Source: CAD feature listing. Evaluate the final solid. Frame: model axes, mm. Face numbers are marked on the shaded views. A direction names the side the tool comes from. Coordinates: 2 decimals unless noted, no trailing zeros. Write each loop counter-clockwise with the first axis right and the second up, starting at its lowest first coordinate (ties: lowest second). Pieces come first, ordered by that corner, then holes. Notation, with made-up numbers: M 79.5,-8 L 122.5,-8 A25 ccw 122.5,19 Z; hole C -7.5,31.5 d2. An arc over 180 degrees is marked long. One line per item, written item: value. Start each with the question number.
Item 1: Cut plane A-A, the plane x = 22. Output: boundary loops of the cut face in (y, z), then the cut area to 3 significant figures.
Item 2: Set-up query: the marked faces 5, 6 and 7. Return all of +Z, -Z, +X, -X, +Y, -Y with unobstructed straight access to the full face (end or side cutting, diameter ignored); none if empty.
Item 3: Mould query, pull axis Y, two halves, no side actions, for the marked faces 1, 2, 3 and 4. Classes: released by +Y, released by -Y, zero draft, split by the parting line, or undercut.
Item 4: Cut plane B-B, the plane y = 35.5. Output: boundary loops of the cut face in (x, z), then the cut area to 3 significant figures.
Item 5: Cut plane C-C, the plane z = 5.5. Output: boundary loops of the cut face in (x, y).
Item 6: Cut plane D-D, the plane x = 56.5. Output: boundary loops of the cut face in (y, z), then the cut area to 3 significant figures.
Item 7: Pin query (flat end, axial travel): P1, Ø17, axis at y = 54.5, z = 25, coming from the -X side; P2, Ø17, axis at y = 22.5, z = 24, coming from the +X side; P3, Ø0.9, axis at x = 102.5, z = 25.5, coming from the +Y side. Return the tip coordinate at first contact, or that it passes through.
Item 8: Ray query, L1, parallel to Y at x = 48, z = 27.5; L2, parallel to X at y = 57, z = 17.5; L3, parallel to Y at x = 16, z = 14.5. Return the intervals inside material, ascending. Write a range as from..to.
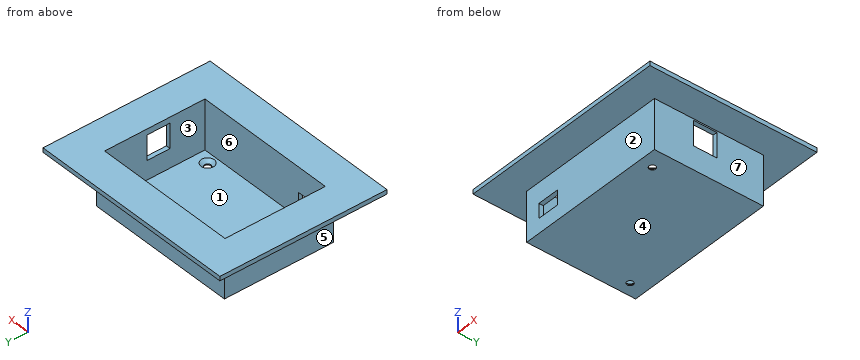
```python
from build123d import *

# Parameters (mm, degrees)
F0_W           = 104
F0_H           = 75
F1_DEPTH       = 37
F2_T           = -3
F4_D           = 4.4
F4_CSINK_D     = 8.96
F4_CSINK_ANGLE = 90
F5_D           = 4.4
F5_CSINK_D     = 8.96
F5_CSINK_ANGLE = 90
F6_W           = 15
F6_H           = 10
F7_DEPTH       = 4
F8_W           = 144
F8_H           = 115
F9_DEPTH       = 3
F10_W          = 98
F10_H          = 69
F11_DEPTH      = 3
F12_W          = 16
F12_H          = 17
F13_DEPTH      = 3


with BuildPart() as f1:
    # F0 (on Top) → F1 (new body)
    with BuildSketch(Plane.XY):
        with Locations((52, 37.5)):
            Rectangle(F0_W, F0_H)
    extrude(amount=F1_DEPTH)

    # F2
    f2_openings = [f1.faces().sort_by_distance(p)[0] for p in [
        (52, 37.5, 37),
    ]]
    offset(amount=F2_T, openings=f2_openings)

    # F4 (through all)
    with Locations(Plane.XY.offset(3)):
        with Locations((8.4720822051, 64.054608345)):
            CounterSinkHole(F4_D / 2, F4_CSINK_D / 2, counter_sink_angle=F4_CSINK_ANGLE)

    # F5 (through all)
    with Locations(Plane.XY.offset(3)):
        with Locations((91.5566533804, 9.1203558259)):
            CounterSinkHole(F5_D / 2, F5_CSINK_D / 2, counter_sink_angle=F5_CSINK_ANGLE)

    # F6 (on face) → F7 (cut)
    with BuildSketch(Plane(origin=(0, 3, 0), x_dir=(-1, 0, 0), z_dir=(0, 1, 0))):
        with Locations((-17.5, 15)):
            Rectangle(F6_W, F6_H)
    extrude(amount=-F7_DEPTH, mode=Mode.SUBTRACT)

    # F8 (on face) → F9 (join)
    with BuildSketch(Plane.XY.offset(37)):
        with Locations((52, 37.5)):
            Rectangle(F8_W, F8_H)
    extrude(amount=-F9_DEPTH)

    # F10 (on face) → F11 (cut)
    with BuildSketch(Plane.XY.offset(37)):
        with Locations((52, 37.5)):
            Rectangle(F10_W, F10_H)
    extrude(amount=-F11_DEPTH, mode=Mode.SUBTRACT)

    # F12 (on face) → F13 (cut)
    with BuildSketch(Plane.YZ.offset(104)):
        with Locations((35, 24.5)):
            Rectangle(F12_W, F12_H)
    extrude(amount=-F13_DEPTH, mode=Mode.SUBTRACT)


solid = f1.part
```
From the geometry:
1. outline: M -20,34 L 0,34 L 0,20 L 3,20 L 3,37 L -20,37 Z; M 0,0 L 75,0 L 75,34 L 95,34 L 95,37 L 72,37 L 72,3 L 3,3 L 3,10 L 0,10 Z
1. area: 519 mm²
2. face 5: -Z, -X, +Y, -Y
2. face 6: +Z
2. face 7: -Z, +X, +Y, -Y
3. face 1: undercut
3. face 2: released by -Y
3. face 3: undercut
3. face 4: zero draft
4. outline: M -20,34 L 0,34 L 0,0 L 104,0 L 104,16 L 101,16 L 101,3 L 3,3 L 3,37 L -20,37 Z; M 101,33 L 104,33 L 104,34 L 124,34 L 124,37 L 101,37 Z
4. area: 585 mm²
5. outline: M 0,0 L 104,0 L 104,75 L 0,75 Z; hole M 3,3 L 101,3 L 101,72 L 3,72 Z
6. outline: M -20,34 L 0,34 L 0,0 L 75,0 L 75,34 L 95,34 L 95,37 L 72,37 L 72,3 L 3,3 L 3,37 L -20,37 Z
6. area: 549 mm²
7. P1: stops at x = 0
7. P2: stops at x = 104
7. P3: stops at y = 75
8. L1: y = 0..3, 72..75
8. L2: x = 0..3, 101..104
8. L3: y = 72..75
